The listing builds one solid part. Answer for the finished solid, in the listing's coordinates (mm). A direction names the side the tool comes from. Give positions to 0.01 mm unless a question says otherwise; leave off trailing zeros. Order: outer loops, then holes, each group sorted by start corner. A loop starts at its lowest first (then second) coordinate and runs counter-clockwise, first axis right, second up.
```python
from build123d import *

# Parameters (mm, degrees)
SALIENTE_EXTRUIR1_DEPTH    = 8.5
CROQUIS2_R                 = 1.25
CORTAR_EXTRUIR1_DEPTH      = 8.5
CROQUIS3_R                 = 3
CORTAR_EXTRUIR2_DEPTH      = 2.5
CORTAR_EXTRUIR3_DEPTH      = 33.009517698
CORTAR_EXTRUIR3_DEPTH_BACK = 33.009517698
CROQUIS4_R                 = 1.5
CROQUIS5_R                 = 3
CORTAR_EXTRUIR4_DEPTH      = 2.5


with BuildPart() as part:
    # Croquis1 → Saliente-Extruir1 (new body)
    with BuildSketch(Plane.XY):
        Polygon((12.15, 8.15), (12.15, 5.65), (10.15, 6.275), (10.15, -6.275), (12.15, -5.65), (12.15, -8.15), (10.15, -7.525), (10.15, -10.15), (15.165647838, -10.15), (15.165647838, 10.15), (10.15, 10.15), (10.15, 7.525), align=None)
    saliente_extruir1 = extrude(amount=SALIENTE_EXTRUIR1_DEPTH)

    # Croquis2 → Cortar-Extruir1 (cut)
    with BuildSketch(Plane.ZY.offset(-10.15)):
        with Locations((4.25, 0)):
            Circle(CROQUIS2_R)
    extrude(amount=-CORTAR_EXTRUIR1_DEPTH, mode=Mode.SUBTRACT)

    # Croquis3 → Cortar-Extruir2 (cut)
    with BuildSketch(Plane.ZY.offset(-10.15)):
        with Locations((4.25, 0)):
            Circle(CROQUIS3_R)
    extrude(amount=-CORTAR_EXTRUIR2_DEPTH, mode=Mode.SUBTRACT)

    # Simetría1: Saliente-Extruir1 across plane
    add(saliente_extruir1.mirror(Plane(origin=(10.15, 10.15, 8.5), x_dir=(0, 0, 1), z_dir=(0, -1, 0))))

    # Croquis4 → Cortar-Extruir3 (cut, two sides: drawn at the far end of the back side and taken through both)
    with BuildSketch(Plane.ZY.offset(-10.15).offset(-CORTAR_EXTRUIR3_DEPTH_BACK)):
        with Locations((4.25, 20.3)):
            Circle(CROQUIS4_R)
    extrude(amount=CORTAR_EXTRUIR3_DEPTH + CORTAR_EXTRUIR3_DEPTH_BACK, mode=Mode.SUBTRACT)

    # Croquis5 → Cortar-Extruir4 (cut)
    with BuildSketch(Plane.ZY.offset(-10.15)):
        with Locations((4.25, 20.3)):
            Circle(CROQUIS5_R)
    extrude(amount=-CORTAR_EXTRUIR4_DEPTH, mode=Mode.SUBTRACT)


solid = part.part
```
1) Find section C-C (z = 4.25). Count the separate pieces of the cut face and the enclosed holes in it, then the cut area to 3 significant figures.
Geometry says:
separate pieces: 3
enclosed holes: 0
area: 145 mm2
2) For a pull along Y with two mould halves and no side action, classify faces 4 (the flat face through (11.136, 12.467, 4.19)), 5 (the flat face through (15.166, 10, 4)), 6 (the flat face through (13, -10.15, 4)) as +Y half, -Y half, draft (parallel to the pull), parting line (faces both ways), or undercut.
Geometry says:
face 4: undercut
face 5: draft
face 6: -Y half
3) Straight lines are drawn through the part: probe 1 along Y at (x, z) = (14.35, 4.25); probe 2 along Y at (x, z) = (12.4, 4.5); probe 3 along X at (y, z) = (20, 1.75). For each, find the intervals that lie inside material, in ascending order.
Geometry says:
probe 1: y = -10.15 to -1.25, 1.25 to 18.8, 21.8 to 30.45
probe 2: y = -10.15 to -2.99, 2.99 to 17.31, 23.29 to 30.45
probe 3: x = 12.65 to 15.17
4) Find section A-A (y = 20.3). Write down the section's boundary in (x, z).
Geometry says:
outline: (10.15, 0) - (15.17, 0) - (15.17, 2.75) - (12.65, 2.75) - (12.65, 1.25) - (10.15, 1.25) - close; (10.15, 7.25) - (12.65, 7.25) - (12.65, 5.75) - (15.17, 5.75) - (15.17, 8.5) - (10.15, 8.5) - close
5) Find section B-B (x = 10.85). Write down the section's boundary in (y, z).
Geometry says:
outline: (-10.15, 0) - (-7.74, 0) - (-7.74, 8.5) - (-10.15, 8.5) - close; (-6.06, 0) - (6.06, 0) - (6.06, 8.5) - (-6.06, 8.5) - close; (7.74, 0) - (12.56, 0) - (12.56, 8.5) - (7.74, 8.5) - close; (14.24, 0) - (26.36, 0) - (26.36, 8.5) - (14.24, 8.5) - close; (28.04, 0) - (30.45, 0) - (30.45, 8.5) - (28.04, 8.5) - close; hole circle Ø6 at (0, 4.25); hole circle Ø6 at (20.3, 4.25)
6) Given P1, Ø4, axis at y = -1.5, z = 5.5, coming from the -X side; P2, Ø3, axis at y = 21, z = 3, coming from the -X side; P3, Ø0.8, axis at y = 7, z = 2.5, coming from the -X side, each flat-ended and moving along its own axis, determine where each tip first touches the part or whether it passes through.
Geometry says:
P1: stops at x = 10.15
P2: stops at x = 12.65
P3: stops at x = 12.15
7) Find section D-D (y = 0). Write down the section's boundary in (x, z).
Geometry says:
outline: (10.15, 0) - (15.17, 0) - (15.17, 3) - (12.65, 3) - (12.65, 1.25) - (10.15, 1.25) - close; (10.15, 7.25) - (12.65, 7.25) - (12.65, 5.5) - (15.17, 5.5) - (15.17, 8.5) - (10.15, 8.5) - close
8) A tool of negligible diameter and unlimited length cuts with its end or side. For faces 1 (the flat face through (11.16, 14.34, 4.19)), 2 (the cylindrical face through (14, 19, 5)), 3 (the cylindrical face through (11.38, 22.33, 2.04)), from which of +Z, -Z, +X, -X, +Y, -Y can it reach the whole face along a straight path? Write none if from no direction.
Geometry says:
face 1: +Z, -Z
face 2: +X, -X
face 3: -X
